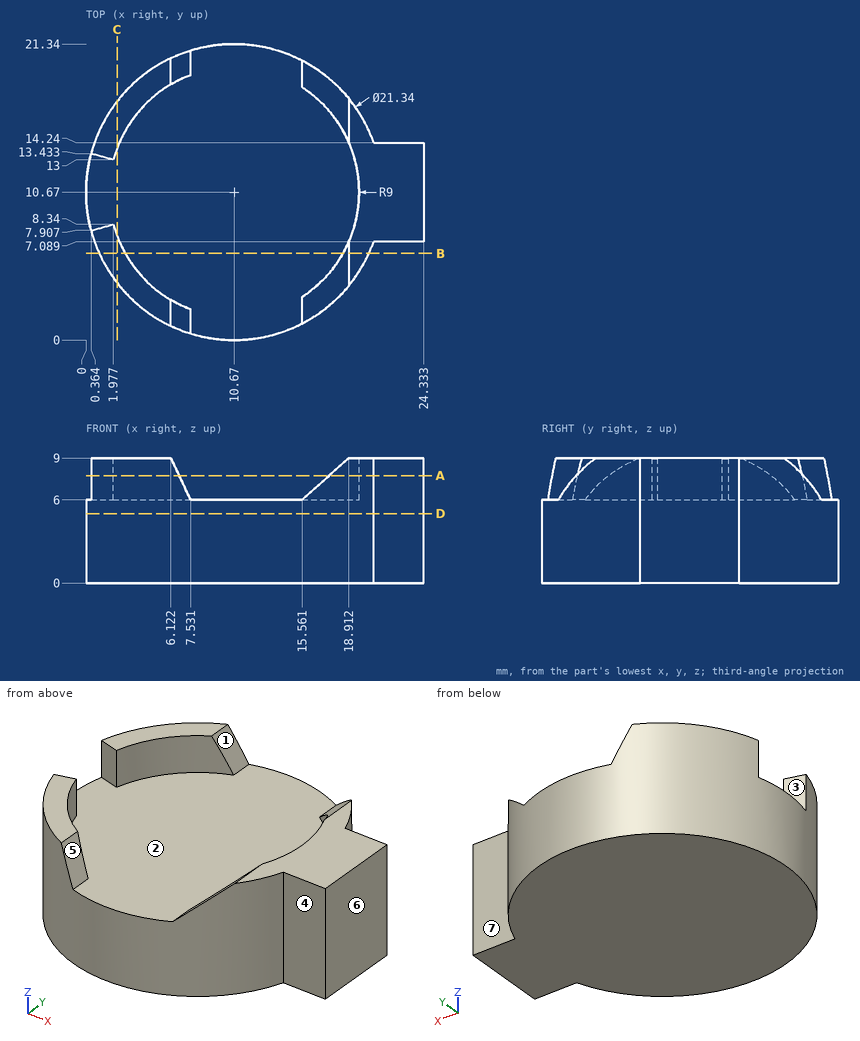
The figure shows three views and two pictorial views of one solid part (mm, origin at its lowest corner). Answer the questions. A direction names the side the tool comes from. Give positions to 0.01 mm unless a question says otherwise; leave off trailing zeros. Write each loop counter-clockwise with the first axis right and the second up, starting at its lowest first coordinate (ties: lowest second). Pieces come first, ordered by that corner, then holes.
Q1. Given pin 1 (3 mm diameter, centred on y = 4.5, z = 4, fed in from -X); pin 2 (6 mm diameter, centred on x = 9, y = 13, fed in from +Z); pin 3 (3 mm diameter, centred on x = 21.5, z = 2.5, fed in from -Y) (1 decimal), each flat-ended and moving along its own axis, determine where each tip first touches the part or whether it passes through.
Answer:
pin 1: stops at x = 1.08
pin 2: stops at z = 6
pin 3: stops at y = 5.5
Q2. The part is cut by section A-A on z = 7.75. Give the vertices of the cut face in (x, y) (1 decimal).
Answer:
outline: (0.4, 7.9) arc R10.7 ccw to (6.7, 0.8) - (6.7, 2.6) arc R9 cw to (2, 8.3) - close; (0.4, 13.4) - (2, 13) arc R9 cw to (6.7, 18.8) - (6.7, 20.6) arc R10.7 ccw to start; (17.5, 2.5) arc R10.7 ccw to (20.7, 7.1) - (24.3, 7.1) - (24.3, 14.2) - (20.7, 14.2) arc R10.7 ccw to (17.5, 18.9) - (17.5, 16.5) arc R9 cw to (17.5, 4.8) - close
Q3. The part is cut by section D-D on z = 5. Give the vertices of the cut face in (x, y) (1 decimal).
Answer:
outline: (20.7, 7.1) - (24.3, 7.1) - (24.3, 14.2) - (20.7, 14.2) arc R10.7 ccw (long way) to start
Q4. A tool of negligible diameter and unlimited length cuts with its end or side. For the marked faces 1, 2, 3 and 4, from which of +Z, -Z, +X, -X, +Y, -Y can it reach the whole face along a straight path? Write none if from no direction.
Answer:
face 1: +Z, +Y, -Y
face 2: +Z
face 3: +Z, -X
face 4: +Z, -Z, +X, -Y
Q5. The part is cut by section B-B on y = 6.25. Give the vertices of the cut face in (x, z).
Answer:
outline: (0.96, 0) - (20.38, 0) - (20.38, 9) - (18.91, 9) - (18.51, 8.64) - (18.51, 6) - (2.83, 6) - (2.83, 9) - (0.96, 9) - close
Q6. Straight lines are drawn through the part: L1, parallel to Z at x = 10, y = 13.5; L2, parallel to X at y = 10.5, z = 3.5; L3, parallel to Y at x = 21.25, z = 5.5. For each, find the intervals that lie inside material, in ascending order.
Answer:
L1: z = 0 to 6
L2: x = 0 to 24.33
L3: y = 7.09 to 14.24
Q7. The part is cut by section C-C on x = 2.25. Give the vertices of the cut face in (y, z), and give its area (3 significant figures).
Answer:
outline: (4.12, 0) - (17.22, 0) - (17.22, 9) - (13.85, 9) - (13.85, 6) - (7.49, 6) - (7.49, 9) - (4.12, 9) - close
area: 98.9 mm2
Q8. For a pull along X with two mould halves and no side action, classify the marked faces 5, 6 and 7 as released by +X, released by -X, zero draft, split by the parting line, or undercut.
Answer:
face 5: undercut
face 6: released by +X
face 7: zero draft
